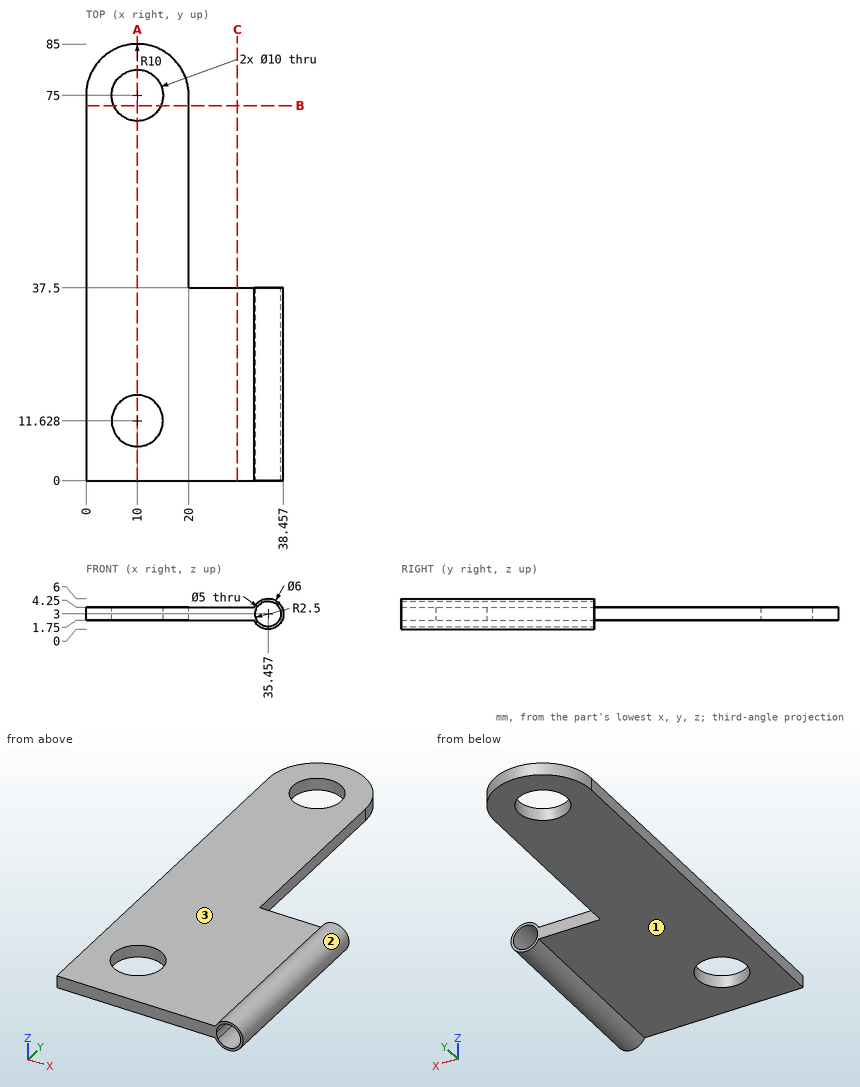
Could you check a few things on this drawing? It's one solid part, dimensions in mm from its lowest x, y, z. A direction names the side the tool comes from. Give positions to 0.01 mm unless a question says otherwise; leave off trailing zeros. Order: outer loops, then holes, each group sorted by start corner. A loop starts at its lowest first (then second) coordinate and runs counter-clockwise, first axis right, second up. Notation, with made-up numbers: (44, -17) - (89, -17) arc R28 cw to (89, 3) - close; hole circle Ø2 at (15, -25). An arc over 180 degrees is marked (long way). One line per item, written item: value. Start each with the question number.
1. Imagine slicing it at A-A on x = 10. List the corners of the cut face in (y, z) for me.
2. For the marked faces 1, 2 and 3, which set-ups out of +Z, -Z, +X, -X, +Y, -Y let a thin tool reach every point of the face, with its end or its side?
3. Imagine slicing it at C-C on x = 29.5. List the corners of the cut face in (y, z) for me.
4. For P1, Ø9, axis at x = 10, y = 75, coming from the +Z side; P2, Ø1.2, axis at y = 48, z = 3.5, coming from the +X side; P3, Ø1, axis at x = 7, y = 41.5, coming from the +Z side, each with a flat end and sliding along its axis, tell me the tip position at first contact or that it passes through.
5. If I drill on probe 1 along Y at (x, z) = (10, 3.2); probe 2 along X at (y, z) = (12, 3); probe 3 along Z at (x, y) = (18.5, 16.5), over which ranges is the centre line in solid material (lowest first)?
6. Imagine slicing it at B-B on y = 73. List the corners of the cut face in (x, z) for me.
Values:
1. outline: (0, 1.75) - (6.63, 1.75) - (6.63, 4.25) - (0, 4.25) - close; (16.63, 1.75) - (70, 1.75) - (70, 4.25) - (16.63, 4.25) - close; (80, 1.75) - (85, 1.75) - (85, 4.25) - (80, 4.25) - close
2. face 1: -Z, -X, +Y, -Y
2. face 2: +Y, -Y
2. face 3: +Z, -X, +Y, -Y
3. outline: (0, 1.75) - (37.5, 1.75) - (37.5, 4.25) - (0, 4.25) - close
4. P1: through
4. P2: x = 20
4. P3: z = 4.25
5. probe 1: 0 to 6.63, 16.63 to 70, 80 to 85
5. probe 2: 0 to 5.01, 14.99 to 32.96, 37.96 to 38.46
5. probe 3: 1.75 to 4.25
6. outline: (0, 1.75) - (5.42, 1.75) - (5.42, 4.25) - (0, 4.25) - close; (14.58, 1.75) - (20, 1.75) - (20, 4.25) - (14.58, 4.25) - close
